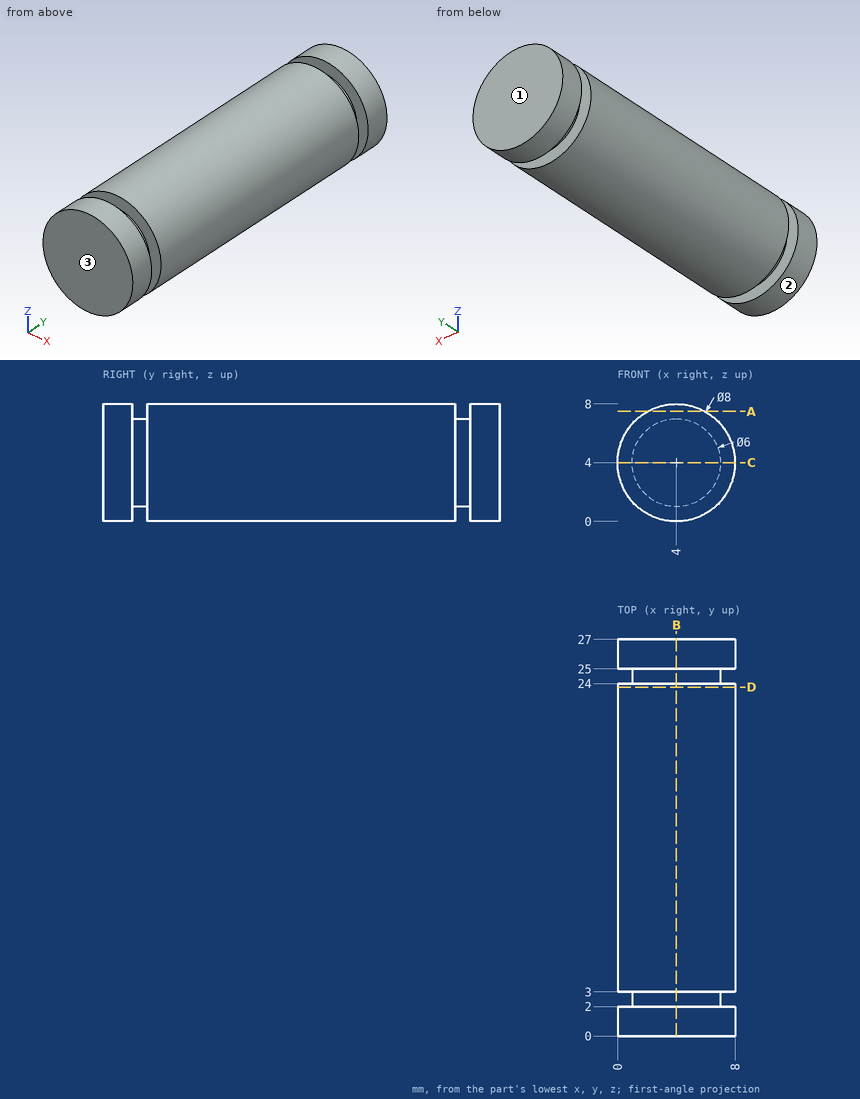
Design review of the part shown in the three views and the two pictorial views. Dimensions are in mm from the part's minimum x, y and z. Round coordinates to 2 decimals unless told otherwise and drop trailing zeros. Loops run counter-clockwise (first coordinate to the right, second up) from the corner with the lowest first, then second, coordinate; pieces in that order, holes last. Notation, with made-up numbers: (79.25, -15.75) - (86.25, -15.75) arc R24 ccw to (86.25, 13.25) - close; hole circle Ø5 at (20.25, 85). An arc over 180 degrees is marked (long way). One line per item, written item: value. Start each with the question number.
Item 1: The part is to be moulded in two halves that separate along Y. For the marked faces 1, 2 and 3, say which applies: +Y half, -Y half, draft (parallel to the pull), parting line (faces both ways), or undercut.
Item 2: Take a section at A-A (z = 7.5). Give the boundary of the cut face in (x, y).
Item 3: For L1, parallel to Y at x = 1.5, z = 2; L2, parallel to Z at x = 1.5, y = 13.75; L3, parallel to Z at x = 3.5, y = 5, list the stretches that pass through material, from the lowest coordinate up.
Item 4: Clearance check with flat-ended pins moving along their axes: pin 1 Ø1.5 at (y, z) = (15, 1) entering from -X; pin 2 Ø3 at (y, z) = (22, 2) entering from -X; pin 3 Ø2 at (y, z) = (10.5, 1) entering from +X. State where each tip first meets the part, or that it passes through.
Item 5: Take a section at B-B (x = 4). Give the boundary of the cut face in (y, z).
Item 6: Take a section at C-C (z = 4). Give the boundary of the cut face in (x, y).
Item 7: Take a section at D-D (y = 23.75). Give the boundary of the cut face in (x, z), plus the area to 3 significant figures.
Answer below:
1. face 1: +Y half
1. face 2: draft
1. face 3: -Y half
2. outline: (2.06, 0) - (5.94, 0) - (5.94, 2) - (2.06, 2) - close; (2.06, 3) - (5.94, 3) - (5.94, 24) - (2.06, 24) - close; (2.06, 25) - (5.94, 25) - (5.94, 27) - (2.06, 27) - close
3. L1: y = 0 to 2, 3 to 24, 25 to 27
3. L2: z = 0.88 to 7.12
3. L3: z = 0.03 to 7.97
4. pin 1: stops at x = 0.69
4. pin 2: stops at x = 0.03
4. pin 3: stops at x = 7.46
5. outline: (0, 0) - (2, 0) - (2, 1) - (3, 1) - (3, 0) - (24, 0) - (24, 1) - (25, 1) - (25, 0) - (27, 0) - (27, 8) - (25, 8) - (25, 7) - (24, 7) - (24, 8) - (3, 8) - (3, 7) - (2, 7) - (2, 8) - (0, 8) - close
6. outline: (0, 0) - (8, 0) - (8, 2) - (7, 2) - (7, 3) - (8, 3) - (8, 24) - (7, 24) - (7, 25) - (8, 25) - (8, 27) - (0, 27) - (0, 25) - (1, 25) - (1, 24) - (0, 24) - (0, 3) - (1, 3) - (1, 2) - (0, 2) - close
7. outline: circle Ø8 at (4, 4)
7. area: 50.3 mm2
